The model under review builds one solid part; all positions refer to its coordinate system, in mm. A direction names the side the tool comes from. Give positions to 0.01 mm unless a question says otherwise; leave off trailing zeros. Loops run counter-clockwise (first coordinate to the right, second up) from the corner with the lowest first, then second, coordinate; pieces in that order, holes last. Notation, with made-up numbers: M 50,55 L 57,55 A16 ccw 57,63 Z; hole C 61.25,50.25 d5. An arc over 180 degrees is marked long. Put each result on its own line as item: value. Start each with the question number.
from build123d import *

# Parameters (mm, degrees)
SM_BASE_FLANGE_1_DEPTH      = 266.5
SM_BASE_FLANGE_1_DEPTH_BACK = 20
EXTRUDE_2_DEPTH             = 5
CUT_EXTRUDE_1_DEPTH         = 781.997587301
SKETCH_16_R                 = 5
CUT_EXTRUDE_6_DEPTH         = 804.201519225
CUT_EXTRUDE_7_DEPTH         = 780.82164677
SKETCH_18_W                 = 41.523044305
SKETCH_18_H                 = 20
SKETCH_18_R                 = 5
CUT_EXTRUDE_8_DEPTH         = 780.82164677
CUT_EXTRUDE_9_DEPTH         = 5
CUT_EXTRUDE_10_DEPTH        = 780.82164677
FILLET_1_R                  = 5
FILLET_2_R                  = 15
FILLET_3_R                  = 5


# Sheet-metal steps are written as plain solids
with BuildPart() as part:
    # Sketch 1 → ﾍﾞｰｽ-ﾌﾗﾝｼﾞ1 (new, two sides: drawn at the far end of the back side and taken through both)
    with BuildSketch(Plane(origin=(0, 0, 0), x_dir=(1, 0, 0), z_dir=(0, 1, 0)).offset(-SM_BASE_FLANGE_1_DEPTH_BACK)):
        with BuildLine():
            Line((137.550775542, 90.408639918), (37.357880769, -9.784254855))
            ThreePointArc((37.357880769, -9.784254855), (37.11891053, -9.943929664), (36.837025914, -10))
            Line((36.837025914, -10), (30, -10))
            Line((30, -10), (-450.5, -10))
            Line((-450.5, -10), (-450.5, -15))
            Line((-450.5, -15), (30, -15))
            Line((30, -15), (36.837025914, -15))
            ThreePointArc((36.837025914, -15), (39.032327692, -14.563327326), (40.893414675, -13.319788761))
            Line((40.893414675, -13.319788761), (141.086309448, 86.873106012))
            Line((141.086309448, 86.873106012), (137.550775542, 90.408639918))
        make_face()
    extrude(amount=SM_BASE_FLANGE_1_DEPTH + SM_BASE_FLANGE_1_DEPTH_BACK)

    # ｽｹｯﾁ15 → ﾎﾞｽ - 押し出し2 (add)
    with BuildSketch(Plane.XY.offset(15)):
        Polygon((-450.5, 0), (-585.5, -486), (-585.5, -506), (124.5, -506), (124.5, -486), (-6, 0), align=None)
    extrude(amount=-EXTRUDE_2_DEPTH)

    # ｽｹｯﾁ7 → ｶｯﾄ - 押し出し1 (cut, through all)
    with BuildSketch(Plane.XY.offset(15)):
        Polygon((-278.755408603, 0), (-151.149515417, 266.5), (-450.5, 266.5), (-450.5, 0), align=None)
    extrude(amount=-CUT_EXTRUDE_1_DEPTH, mode=Mode.SUBTRACT)

    # ｽｹｯﾁ16 → ｶｯﾄ - 押し出し6 (cut, through all)
    with BuildSketch(Plane(origin=(27.106601718, 0, 27.106601718), x_dir=(0.7071067811865438, 0, -0.7071067811865513), z_dir=(0.7071067811865513, 0, 0.7071067811865438))):
        with BuildLine():
            Line((23.323748893, 266.5), (148.323748893, 0))
            Line((148.323748893, 0), (136.191648507, 0))
            ThreePointArc((136.191648507, 0), (132.656114601, -1.464466094), (131.191648507, -5))
            Line((131.191648507, -5), (131.191648507, -20))
            Line((131.191648507, -20), (141.191648507, -20))
            Line((141.191648507, -20), (161.191648507, -20))
            Line((161.191648507, -20), (161.191648507, 266.5))
            Line((161.191648507, 266.5), (23.323748893, 266.5))
        make_face()
        with BuildLine():
            Line((51.191648507, 0), (19.497497865, 0))
            Line((19.497497865, 0), (19.497497865, -20))
            Line((19.497497865, -20), (46.191648507, -20))
            Line((46.191648507, -20), (56.191648507, -20))
            Line((56.191648507, -20), (56.191648507, -5))
            ThreePointArc((56.191648507, -5), (54.727182413, -1.464466094), (51.191648507, 0))
        make_face()
        with Locations(Location((116.191648507, -10, 0), (0, 0, 180))):
            Circle(SKETCH_16_R)
        with Locations(Location((71.191648507, -10, 0), (0, 0, 180))):
            Circle(SKETCH_16_R)
    extrude(amount=-CUT_EXTRUDE_6_DEPTH, mode=Mode.SUBTRACT)

    # ｽｹｯﾁ17 → ｶｯﾄ - 押し出し7 (cut, through all)
    with BuildSketch(Plane.XY.offset(15)):
        with BuildLine():
            Line((-416.055555556, -20), (-316.055555556, -20))
            ThreePointArc((-316.055555556, -20), (-301.055555556, -35), (-316.055555556, -50))
            Line((-316.055555556, -50), (-416.055555556, -50))
            ThreePointArc((-416.055555556, -50), (-431.055555556, -35), (-416.055555556, -20))
        make_face()
    extrude(amount=-CUT_EXTRUDE_7_DEPTH, mode=Mode.SUBTRACT)

    # ｽｹｯﾁ18 → ｶｯﾄ - 押し出し8 (cut, through all)
    with BuildSketch(Plane.XY.offset(15)):
        with BuildLine():
            Line((-78, -5), (-118, -5))
            ThreePointArc((-118, -5), (-123, -10), (-118, -15))
            Line((-118, -15), (-78, -15))
            ThreePointArc((-78, -15), (-73, -10), (-78, -5))
        make_face()
        with BuildLine():
            Line((-123, 266.5), (-123, 261.5))
            ThreePointArc((-123, 261.5), (-121.535533906, 257.964466094), (-118, 256.5))
            Line((-118, 256.5), (-78, 256.5))
            ThreePointArc((-78, 256.5), (-74.464466094, 257.964466094), (-73, 261.5))
            Line((-73, 261.5), (-73, 266.5))
            Line((-73, 266.5), (-123, 266.5))
        make_face()
        with BuildLine():
            ThreePointArc((0, 261.5), (1.464466094, 257.964466094), (5, 256.5))
            Line((5, 256.5), (25, 256.5))
            ThreePointArc((25, 256.5), (28.535533906, 257.964466094), (30, 261.5))
            Line((30, 261.5), (30, 266.5))
            Line((30, 266.5), (0, 266.5))
            Line((0, 266.5), (0, 261.5))
        make_face()
        with BuildLine():
            Line((-143, 266.5), (-151.149515417, 266.5))
            Line((-151.149515417, 266.5), (-155.937729045, 256.5))
            Line((-155.937729045, 256.5), (-148, 256.5))
            ThreePointArc((-148, 256.5), (-144.464466094, 257.964466094), (-143, 261.5))
            Line((-143, 261.5), (-143, 266.5))
        make_face()
        with Locations((20.131892523, -10)):
            Rectangle(SKETCH_18_W, SKETCH_18_H)
        with Locations(Location((110, -496, 0), (0, 0, 180))):
            Circle(SKETCH_18_R)
        with Locations(Location((-571, -496, 0), (0, 0, 180))):
            Circle(SKETCH_18_R)
        with Locations(Location((-213, -496, 0), (0, 0, 180))):
            Circle(SKETCH_18_R)
        with Locations(Location((-248, -496, 0), (0, 0, 180))):
            Circle(SKETCH_18_R)
        with Locations(Location((-440.5, -10, 0), (0, 0, 180))):
            Circle(SKETCH_18_R)
        with Locations(Location((-20.5, -10, 0), (0, 0, 180))):
            Circle(SKETCH_18_R)
        with Locations(Location((-278, -10, 0), (0, 0, 180))):
            Circle(SKETCH_18_R)
    extrude(amount=-CUT_EXTRUDE_8_DEPTH, mode=Mode.SUBTRACT)

    # ｽｹｯﾁ24 → ｶｯﾄ - 押し出し9 (cut)
    with BuildSketch(Plane.XY.offset(15)):
        with BuildLine():
            ThreePointArc((-337, -238.291287847), (-338, -233.5), (-339, -238.291287847))
            Line((-339, -238.291287847), (-339, -486))
            Line((-339, -486), (-122, -486))
            Line((-122, -486), (-122, -238.291287847))
            ThreePointArc((-122, -238.291287847), (-123, -233.5), (-124, -238.291287847))
            Line((-124, -238.291287847), (-124, -484))
            Line((-124, -484), (-337, -484))
            Line((-337, -484), (-337, -238.291287847))
        make_face()
    extrude(amount=-CUT_EXTRUDE_9_DEPTH, mode=Mode.SUBTRACT)

    # ｽｹｯﾁ25 → ｶｯﾄ - 押し出し10 (cut, through all)
    with BuildSketch(Plane.XY.offset(15)):
        Polygon((-44.345258018, -50), (-72, -50), (-72, -238.291287847), (6.214439645, -238.291287847), align=None)
        Polygon((-389, -238.291287847), (-389, -100), (-426.38460641, -100), (-464.798853035, -238.291287847), align=None)
    extrude(amount=-CUT_EXTRUDE_10_DEPTH, mode=Mode.SUBTRACT)

    # ﾌｨﾚｯﾄ1
    fillet_1_edges = [part.edges().sort_by_distance(p)[0] for p in [
        (-0.62962963, 0, 12.5),
    ]]
    fillet(fillet_1_edges, radius=FILLET_1_R)

    # ﾌｨﾚｯﾄ2
    fillet_2_edges = [part.edges().sort_by_distance(p)[0] for p in [
        (-389, -238.291287847, 12.5),
        (-464.798853035, -238.291287847, 12.5),
        (-426.38460641, -100, 12.5),
        (-389, -100, 12.5),
        (-72, -238.291287847, 12.5),
        (-72, -50, 12.5),
        (-44.345258018, -50, 12.5),
        (6.214439645, -238.291287847, 12.5),
    ]]
    fillet(fillet_2_edges, radius=FILLET_2_R)

    # ﾌｨﾚｯﾄ3
    fillet_3_edges = [part.edges().sort_by_distance(p)[0] for p in [
        (-155.937729045, 256.5, 12.5),
        (-143, 266.5, 12.5),
        (-123, 266.5, 12.5),
        (-73, 266.5, 12.5),
        (0, 266.5, 12.5),
        (30, 266.5, 12.5),
        (41.831215769, 266.5, 8.84645376),
        (130.219563418, 0, -79.541893888),
        (118.105339059, -20, -67.42766953),
        (65.07233047, -20, -14.394660941),
        (124.5, -486, 12.5),
        (124.5, -506, 12.5),
        (-585.5, -506, 12.5),
        (-585.5, -486, 12.5),
        (-450.5, 0, 12.5),
        (-278.755408603, 0, 12.5),
    ]]
    fillet(fillet_3_edges, radius=FILLET_3_R - 0.0001)  # a hair under: the kernel refuses the full size


solid = part.part
(1) Insertion check: pin 1 (2.5 mm diameter, centred on x = -97, z = 13.5, fed in from +Y); pin 2 (4 mm diameter, centred on y = -347, z = 13, fed in from -X); pin 3 (4 mm diameter, centred on x = -356, z = 13.5, fed in from +Y); pin 4 (9 mm diameter, centred on x = -440.5, y = -10, fed in from -Z). Each pin has a flat end and moves straight along its axis. Give the tip position at first contact, or say it passes through.
(2) We need section D-D, the plane x = -472. Write out the cut boundary in (y, z), plus the area to 3 significant figures.
(3) We need section B-B, the plane y = -35. Write out the cut boundary in (x, z), plus the area to 3 significant figures.
(4) We need section A-A, the plane y = -343.5. Write out the cut boundary in (x, z), plus the area to 3 significant figures.
(5) To check wall thickness, follow L1, parallel to Y at x = -338, z = 11.45; L2, parallel to X at y = -496, z = 11; L3, parallel to X at y = -236, z = 13. State the ranges of each line that lie inside material, in increasing order. Write a range as [from, to].
(6) For faces 4 (the flat face through (-517.48, -241.13, 12.54)), 5 (the flat face through (-444.266, -164.373, 12.535)), 6 (the flat face through (62.724, -255.939, 12.535)), list the 3-axis set-ups (+Z, -Z, +X, -X, +Y, -Y) from which the entire face can be reached by the end or side of a thin tool; tool diameter is ignored.
(7) We need section C-C, the plane x = -179. Write out the cut boundary in (y, z).
(8) Draft analysis for pull direction Y (two halves, no side actions). For faces 1 (the flat face through (-218.19, 126.49, 12.54)), 2 (the flat face through (74.907, 89.411, -20.694)), 3 (the flat face through (-19.812, -141.364, 12.535)), state which applies: +Y half, -Y half, draft (parallel to the pull), parting line (faces both ways), or undercut.
Check sheet entries:
1. pin 1: stops at y = 256.5
1. pin 2: stops at x = -547.44
1. pin 3: stops at y = 0
1. pin 4: passes through
2. outline: M -506,10 L -77.4,10 L -77.4,15 L -506,15 Z
2. area: 2,140 mm²
3. outline: M -460.22,10 L -431.06,10 L -431.06,15 L -460.22,15 Z; M -301.06,10 L 3.4,10 L 3.4,15 L -301.06,15 Z
3. area: 1,670 mm²
4. outline: M -545.92,10 L -339,10 L -339,15 L -545.92,15 Z; M -337,10 L -124,10 L -124,15 L -337,15 Z; M -122,10 L 86.24,10 L 86.24,15 L -122,15 Z
4. area: 3,140 mm²
5. L1: y = [-506, -486], [-233.5, -50], [-20, 0]
5. L2: x = [-585.5, -576], [-566, -253], [-243, -218], [-208, 105], [115, 124.5]
5. L3: x = [-516.06, -453.03], [-396.03, -340.5], [-335.5, -125.5], [-120.5, -64.97], [-5.38, 57.37]
6. face 4: +Z, -Z, -X, +Y
6. face 5: +Z, -Z
6. face 6: +Z, -Z, +X
7. outline: M -506,10 L -486,10 L -486,15 L -506,15 Z; M -484,10 L 208.34,10 L 208.34,15 L -484,15 Z
8. face 1: +Y half
8. face 2: draft
8. face 3: undercut
